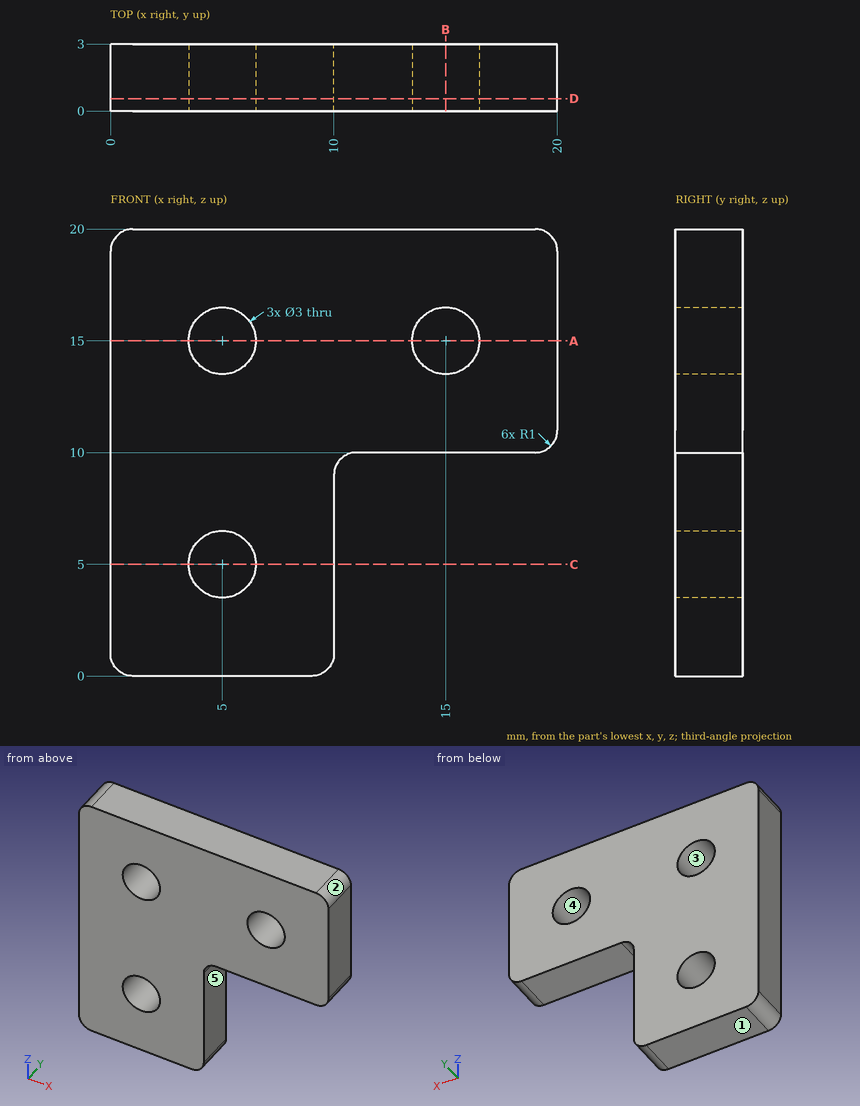
Could you check a few things on this drawing? It's one solid part, dimensions in mm from its lowest x, y, z. A direction names the side the tool comes from. Give positions to 0.01 mm unless a question says otherwise; leave off trailing zeros. Order: outer loops, then holes, each group sorted by start corner. A loop starts at its lowest first (then second) coordinate and runs counter-clockwise, first axis right, second up. Notation, with made-up numbers: M 15.5,82 L 70.5,82 A18 cw 70.5,111 Z; hole C 40.25,14.25 d8. An arc over 180 degrees is marked long. Use one line per item in the form item = value. Start each with the question number.
Item 1: If we section it at B-B (x = 15): Write out the boundary of the cut face in (y, z), then the cut area to 3 significant figures.
Item 2: Will these pins go through, and if not, where does the flat tip stop? pin 1 Ø0.9 at (x, y) = (17, 1) entering from -Z; pin 2 Ø1.8 at (x, z) = (5, 15) entering from +Y.
Item 3: If we section it at A-A (z = 15): Write out the boundary of the cut face in (x, y), then the cut area to 3 significant figures.
Item 4: If we section it at D-D (y = 0.55): Write out the boundary of the cut face in (x, z), then the cut area to 3 significant figures.
Item 5: We'd pull the mould along X, two halves only. Please class the marked faces 1, 2 and 3: +X half, -X half, draft (parallel to the pull), parting line (faces both ways), or undercut.
Item 6: For the marked faces 4 and 5, which set-ups out of +Z, -Z, +X, -X, +Y, -Y let a thin tool reach every point of the face, with its end or its side?
Item 7: If I drill on line 1 along X through (y, z) = (2.1, 15); line 2 along Z through (x, y) = (5.75, 2.7); line 3 along Z through (x, y) = (12, 2.25), over which ranges is the centre line in solid material (lowest first)?
Item 8: If we section it at C-C (z = 5): Write out the boundary of the cut face in (x, y).
Outcome:
q1.outline = M 0,10 L 3,10 L 3,13.5 L 0,13.5 Z; M 0,16.5 L 3,16.5 L 3,20 L 0,20 Z
q1.area = 21.0 mm2
q2.pin_1 = 10
q2.pin_2 = through
q3.outline = M 0,0 L 3.5,0 L 3.5,3 L 0,3 Z; M 6.5,0 L 13.5,0 L 13.5,3 L 6.5,3 Z; M 16.5,0 L 20,0 L 20,3 L 16.5,3 Z
q3.area = 42.0 mm2
q4.outline = M 0,1 A1 ccw 1,0 L 9,0 A1 ccw 10,1 L 10,9 A1 cw 11,10 L 19,10 A1 ccw 20,11 L 20,19 A1 ccw 19,20 L 1,20 A1 ccw 0,19 Z; hole C 5,5 d3; hole C 5,15 d3; hole C 15,15 d3
q4.area = 278 mm2
q5.face_1 = draft
q5.face_2 = +X half
q5.face_3 = undercut
q6.face_4 = +Y, -Y
q6.face_5 = -Z, +X, +Y, -Y
q7.line_1 = 0 to 3.5, 6.5 to 13.5, 16.5 to 20
q7.line_2 = 0 to 3.7, 6.3 to 13.7, 16.3 to 20
q7.line_3 = 10 to 20
q8.outline = M 0,0 L 3.5,0 L 3.5,3 L 0,3 Z; M 6.5,0 L 10,0 L 10,3 L 6.5,3 Z
